```python
from build123d import *

# Parameters (mm, degrees)
PAD020_DEPTH     = 18.5
POCKET047_DEPTH  = 13
POCKET048_DEPTH  = 5
POCKET049_DEPTH  = 15
SKETCH088_R      = 2.75
POCKET050_DEPTH  = 12
SKETCH089_R      = 1.7
POCKET051_DEPTH  = 5
CHAMFER_SIZE     = 3
CHAMFER036_SIZE2 = 3
CHAMFER036_SIZE  = 10
CHAMFER037_SIZE2 = 10
CHAMFER037_SIZE  = 3
CHAMFER038_SIZE  = 1
CHAMFER039_SIZE  = 1
CHAMFER040_SIZE  = 1.5
CHAMFER041_SIZE  = 1
CHAMFER042_SIZE  = 1
CHAMFER043_SIZE  = 1
CHAMFER044_SIZE  = 1
CHAMFER045_SIZE  = 1.5
CHAMFER046_SIZE  = 1
CHAMFER047_SIZE  = 1
CHAMFER048_SIZE  = 1.5
CHAMFER049_SIZE  = 1
CHAMFER050_SIZE  = 1


with BuildPart() as part:
    # Sketch084 → Pad020 (new body)
    with BuildSketch(Plane.XY):
        Polygon((0, 38.8), (8, 38.8), (8, 40.6), (14, 40.6), (14, 38.8), (28, 38.8), (28, 40.6), (34, 40.6), (34, 38.7761214391), (37.3, 38.7761214391), (41.9953022309, 33.1864759261), (38.7027713123, 30.4207499545), (37.673663974, 31.6458777382), (31.9308774881, 26.82193709), (30.0013012288, 29.1190516844), (5.1924636096, 8.2796280843), (7.1220398689, 5.9825134899), (0, 0), align=None)
        Polygon((7.5, 32.8), (7.5, 18.1), (25, 32.8), align=None, mode=Mode.SUBTRACT)
    extrude(amount=PAD020_DEPTH)

    # Sketch085 → Pocket047 (cut)
    with BuildSketch(Plane.XY.offset(6.5)):
        Polygon((0, 5.9744797055), (4.1823490341, 9.4838872374), (7.132775333, 5.967706096), (31.9875690904, 26.8233543707), (29.8491428651, 29.3718315072), (38.9102049805, 36.9749653863), (34.8909759819, 41.7648959848), (21, 41.7648959848), (21, 32.458794), (1, 32.458794), (1, 41.759258), (0, 41.764896), align=None)
    extrude(amount=POCKET047_DEPTH, mode=Mode.SUBTRACT)

    # Sketch086 → Pocket048 (cut)
    with BuildSketch(Plane.XY.offset(16.5)):
        Polygon((-0.8541061726, -4.3526620467), (49.194970654, 37.6434998606), (44.0526697777, 43.7718554052), (-5.9964070501, 1.7756934982), align=None)
    extrude(amount=POCKET048_DEPTH, mode=Mode.SUBTRACT)

    # Sketch087 → Pocket049 (cut)
    with BuildSketch(Plane.XY.offset(5.8)):
        Polygon((37.0972154509, 31.1536445146), (41.470166846, 34.8229864174), (44.3478623025, 31.3934825187), (39.9749109074, 27.724140616), align=None)
        Polygon((6.1, 34.25), (16.1, 34.25), (16.9452365235, 32.4373844259), (5.2547634765, 32.4373844259), align=None)
    extrude(amount=POCKET049_DEPTH, mode=Mode.SUBTRACT)

    # Sketch088 → Pocket050 (cut)
    with BuildSketch(Plane.XZ.offset(-30)):
        with Locations((11.1, 12.9)):
            Circle(SKETCH088_R)
    extrude(amount=-POCKET050_DEPTH, mode=Mode.SUBTRACT)

    # Sketch089 → Pocket051 (cut)
    with BuildSketch(Plane(origin=(0, 0, 0), x_dir=(0.7657048648, 0.6431920864, 0), z_dir=(0.6431920864, -0.7657048648, 0))):
        with Locations((5, 10.6)):
            Circle(SKETCH089_R)
        with Locations((46, 10.6)):
            Circle(SKETCH089_R)
    extrude(amount=-POCKET051_DEPTH, mode=Mode.SUBTRACT)

    # Chamfer
    chamfer_edges = [part.edges().sort_by_distance(p)[0] for p in [
        (39.912516, 35.665983, 16.5),
    ]]
    chamfer(chamfer_edges, length=CHAMFER_SIZE)

    # Chamfer036
    chamfer036_edges = [part.edges().sort_by_distance(p)[0] for p in [
        (21, 35.8, 18.5),
    ]]
    chamfer036_side = part.faces().sort_by_distance((21, 35.8, 12.5))[0]
    chamfer(chamfer036_edges, length=CHAMFER036_SIZE, length2=CHAMFER036_SIZE2, reference=chamfer036_side)

    # Chamfer037
    chamfer037_edges = [part.edges().sort_by_distance(p)[0] for p in [
        (1, 35.629397, 18.5),
    ]]
    chamfer037_side = part.faces().sort_by_distance((9.318343, 36.537604, 18.5))[0]
    chamfer(chamfer037_edges, length=CHAMFER037_SIZE, length2=CHAMFER037_SIZE2, reference=chamfer037_side)

    # Chamfer038
    chamfer038_edges = [part.edges().sort_by_distance(p)[0] for p in [
        (16.25, 25.45, 6.5),
        (7.5, 25.268692, 6.5),
        (23, 32.8, 6.5),
    ]]
    chamfer(chamfer038_edges, length=CHAMFER038_SIZE)

    # Chamfer039
    chamfer039_edges = [part.edges().sort_by_distance(p)[0] for p in [
        (17.388073, 32.8, 18.5),
        (4.632373, 32.458794, 18.5),
    ]]
    chamfer(chamfer039_edges, length=CHAMFER039_SIZE)

    # Chamfer040
    chamfer040_edges = [part.edges().sort_by_distance(p)[0] for p in [
        (31, 40.6, 6.5),
        (11, 40.6, 18.5),
    ]]
    chamfer(chamfer040_edges, length=CHAMFER040_SIZE)

    # Chamfer041
    chamfer041_edges = [part.edges().sort_by_distance(p)[0] for p in [
        (38.076586, 37.851615, 6.5),
    ]]
    chamfer(chamfer041_edges, length=CHAMFER041_SIZE)

    # Chamfer042
    chamfer042_edges = [part.edges().sort_by_distance(p)[0] for p in [
        (0, 22.38724, 6.5),
        (0, 19.4, 0),
    ]]
    chamfer(chamfer042_edges, length=CHAMFER042_SIZE)

    # Chamfer043
    chamfer043_edges = [part.edges().sort_by_distance(p)[0] for p in [
        (0, 38.8, 3.25),
    ]]
    chamfer(chamfer043_edges, length=CHAMFER043_SIZE)

    # Chamfer044
    chamfer044_edges = [part.edges().sort_by_distance(p)[0] for p in [
        (0, 0, 8.75),
    ]]
    chamfer(chamfer044_edges, length=CHAMFER044_SIZE)

    # Chamfer045
    chamfer045_edges = [part.edges().sort_by_distance(p)[0] for p in [
        (2.091175, 7.729183, 16.5),
        (0, 3.48724, 16.5),
    ]]
    chamfer(chamfer045_edges, length=CHAMFER045_SIZE)

    # Chamfer046
    chamfer046_edges = [part.edges().sort_by_distance(p)[0] for p in [
        (1.132852, 0.951596, 16.132852),
    ]]
    chamfer(chamfer046_edges, length=CHAMFER046_SIZE)

    # Chamfer047
    chamfer047_edges = [part.edges().sort_by_distance(p)[0] for p in [
        (16.25, 25.45, 0),
        (16.25, 32.8, 0),
        (7.5, 25.45, 0),
    ]]
    chamfer(chamfer047_edges, length=CHAMFER047_SIZE)

    # Chamfer048
    chamfer048_edges = [part.edges().sort_by_distance(p)[0] for p in [
        (4.06102, 3.411257, 0),
        (17.596882, 18.69934, 0),
        (34.802271, 29.233907, 0),
    ]]
    chamfer(chamfer048_edges, length=CHAMFER048_SIZE)

    # Chamfer049
    chamfer049_edges = [part.edges().sort_by_distance(p)[0] for p in [
        (30.483695, 28.544773, 0),
        (29.518907, 29.69333, 0),
    ]]
    chamfer(chamfer049_edges, length=CHAMFER049_SIZE)

    # Chamfer050
    chamfer050_edges = [part.edges().sort_by_distance(p)[0] for p in [
        (4.71007, 8.853907, 0),
    ]]
    chamfer(chamfer050_edges, length=CHAMFER050_SIZE)


with BuildPart() as part_1:
    # Body016 placement: moved
    add(part.part.moved(Location((57, 0, 0))))


solid = part_1.part
```
Can you work these out from the model? Positions are in its coordinate system, mm. A direction names the side the tool comes from. Give positions to 0.01 mm unless a question says otherwise; leave off trailing zeros. Loops run counter-clockwise (first coordinate to the right, second up) from the corner with the lowest first, then second, coordinate; pieces in that order, holes last. Notation, with made-up numbers: M 33.25,86 L 71.25,86 A18 ccw 71.25,90 Z; hole C 11,1.25 d11. An arc over 180 degrees is marked long. Use CSV: the item, a comma, the result in double quotes. Start each with the question number.
1. Imagine slicing it at C-C, the plane x = 68.1. Write out the boundary of the cut face in (y, z), plus the area to 3 significant figures.
2. Imagine slicing it at D-D, the plane y = 35.5. Write out the boundary of the cut face in (x, z).
3. Imagine slicing it at B-B, the plane y = 22.5. Write out the boundary of the cut face in (x, z).
4. Imagine slicing it at A-A, the plane z = 12.9. Count the separate pieces of the cut face and the enclosed holes in it, plus the area to 3 significant figures.
5. If I drill on L1, parallel to Z at x = 68.1, y = 38.25; L2, parallel to Y at x = 76, z = 3.75; L3, parallel to Y at x = 67, z = 7.5, over which ranges is the centre line in solid material (lowest first)?
6. On a 3-axis mill with a long thin cutter (end or side, diameter ignored), from which of +Z, -Z, +X, -X, +Y, -Y can I reach the whole of each face in a straight line? I mean faces 1 (the face through (80.7, 33.3, 6)), 2 (the face through (91.29, 33.1, 12.15)), 3 (the face through (91, 40, 3)). Say none if no direction works.
7. If we mould it in two halves opening along X, with no side actions, what happens to faces 4 (the face through (61, 38.8, 9)), 5 (the face through (95.73, 34.71, 15.02)), 6 (the face through (73, 32.8, 5)), 7 (the face through (71, 40, 9))? For each: released by +X, released by -X, zero draft, split by the parting line, or undercut.
8. For P1, Ø1.5, axis at y = 27, z = 16.5, coming from the -X side; P2, Ø1.2, axis at x = 97, y = 33, coming from the +Z side; P3, Ø5, axis at y = 29, z = 9, coming from the +X side, each with a flat end and sliding along its axis, tell me the tip position at first contact or that it passes through.
Response values:
1,outline,"M 13.24,1.5 L 15.2,0 L 19.82,0 L 21.12,1 L 21.12,5.5 L 19.82,6.5 L 13.24,6.5 Z; M 32.8,1 L 33.8,0 L 40.6,0 L 40.6,10.15 L 34.25,10.15 L 34.25,5.8 L 32.8,5.8 Z; M 34.25,15.65 L 40.6,15.65 L 40.6,17 L 39.1,18.5 L 34.25,18.5 Z"
1,area,"138 mm^2"
2,outline,"M 57,1 L 58,0 L 97.05,0 L 97.05,13.5 L 94.15,15.72 L 94.15,6.5 L 78,6.5 L 78,8.5 L 75,18.5 L 61,18.5 L 58,8.5 L 58,6.5 L 57,5.5 Z; hole C 68.1,12.9 d5.5"
3,outline,"M 57,1 L 58,0 L 63.5,0 L 64.5,1 L 64.5,5.5 L 63.5,6.5 L 58,6.5 L 57,5.5 Z; M 69.74,1 L 71.29,0 L 76.79,0 L 79.12,1.5 L 79.12,6.5 L 71.29,6.5 L 69.74,5.5 Z"
4,separate pieces,"4"
4,enclosed holes,"0"
4,area,"138 mm^2"
5,L1,"0 to 10.15, 15.65 to 18.5"
5,L2,"19.88 to 27.76, 32.8 to 38.8"
5,L3,"34.25 to 40.6"
6,face 1,"+Z"
6,face 2,"+Z, +Y"
6,face 3,"+Z, -Z, +X, +Y"
7,face 4,"zero draft"
7,face 5,"released by +X"
7,face 6,"undercut"
7,face 7,"undercut"
8,P1,"x = 88.21"
8,P2,"z = 15.54"
8,P3,"x = 94.5"
